Design review of the part shown in the three views and the two pictorial views. Dimensions are in mm from the part's minimum x, y and z. Give positions to 0.01 mm unless a question says otherwise; leave off trailing zeros. Order: outer loops, then holes, each group sorted by start corner. A loop starts at its lowest first (then second) coordinate and runs counter-clockwise, first axis right, second up. Notation, with made-up numbers: (-13, 35) - (16, 35) arc R32 cw to (16, 72) - close; hole circle Ø8 at (63.5, 82.5). An arc over 180 degrees is marked (long way). Put each result on its own line as item: value. Start each with the question number.
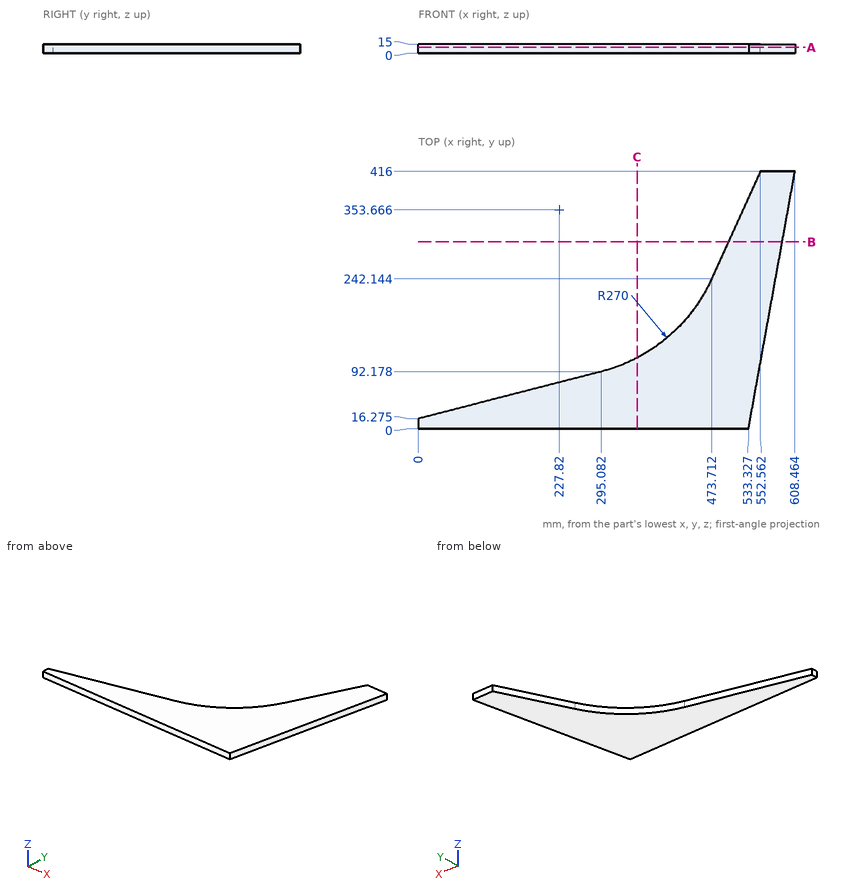
1. Clearance check with flat-ended pins moving along their axes: pin 1 (5 mm diameter, centred on y = 116, z = 6, fed in from +X); pin 2 (5 mm diameter, centred on x = 259, z = 12, fed in from +Y); pin 3 (1.5 mm diameter, centred on x = 461.5, z = 3.5, fed in from +Y) (1 decimal). State where each tip first meets the part, or that it passes through.
2. Add section A-A, the plane z = 9.5. Give the boundary of the cut face in (x, y) (1 decimal).
3. Wall thickness on line 1 (Y direction, x = 295.5, z = 8.25) (1 decimal); line 2 (X direction, y = 238, z = 5) (1 decimal); line 3 (Y direction, x = 467, z = 8.5) (1 decimal): over which ranges is each line inside the solid? List them lowest first. Write a range as from..to.
4. Add section B-B, the plane y = 302. Give the boundary of the cut face in (x, z).
5. Add section C-C, the plane x = 353.5. Give the boundary of the cut face in (y, z).
Found:
1. pin 1: stops at x = 554.73
1. pin 2: stops at y = 83.54
1. pin 3: stops at y = 219.7
2. outline: (0, 0) - (533.3, 0) - (608.5, 416) - (552.6, 416) - (473.7, 242.1) arc R270 cw to (295.1, 92.2) - (0, 16.3) - close
3. line 1: y = 0..92.3
3. line 2: x = 471.8..576.3
3. line 3: y = 0..228.4
4. outline: (500.86, 0) - (587.87, 0) - (587.87, 15) - (500.86, 15) - close
5. outline: (0, 0) - (114.7, 0) - (114.7, 15) - (0, 15) - close
